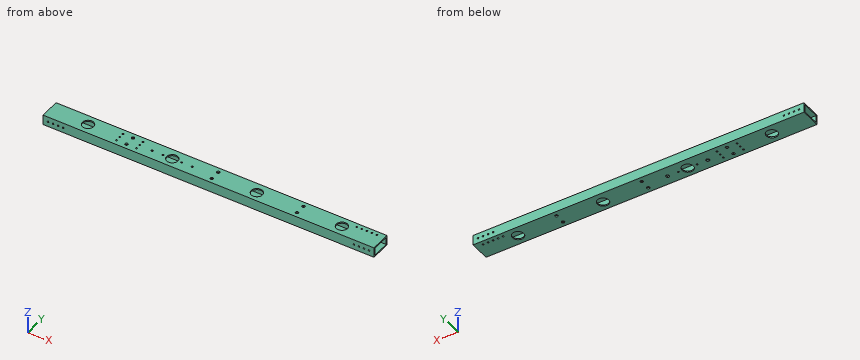
Autodesk Inventor part; units mm, degrees
ref_plane "YZ Plane" through (0, 0, 0) normal (1, 0, 0) x (0, 1, 0)
ref_plane "XZ Plane" through (0, 0, 0) normal (0, 1, 0) x (-1, 0, 0)
ref_plane "XY Plane" through (0, 0, 0) normal (0, 0, 1) x (1, 0, 0)
sketch "Sketch1" plane through (0, 0, 0) normal (0, 1, 0) x (-1, 0, 0)
  point P0 (0, 0)
sketch "Sketch2" plane through (0, 0, 0) normal (0, 0, 1) x (1, 0, 0)
  line L0 (0, 0) -> (838.2, 0)
  line L1 (838.2, 0) -> (838.2, 50.8)
  line L2 (838.2, 50.8) -> (0, 50.8)
  line L3 (0, 50.8) -> (0, 0)
  circle A0 centre (740.5688, 25.4) radius 14.2875
  circle A1 centre (97.6371, 25.4) radius 14.2875
  line L4 (0, 25.4) -> (838.2, 25.4) construction
  circle A2 centre (311.9438, 23.8125) radius 14.2875
  circle A3 centre (288.1313, 23.8125) radius 2.159
  circle A4 centre (335.7563, 23.8125) radius 2.159
  circle A5 centre (362.7438, 23.8125) radius 2.54
  circle A6 centre (261.1438, 23.8125) radius 2.54
  circle A7 centre (327.8188, 23.8125) radius 7.9375 construction
  line L5 (97.6371, 25.4) -> (97.6371, 90.8259)
  line L6 (740.5688, 25.4) -> (740.5688, 86.7676)
  line L7 (327.8188, 23.8125) -> (327.8188, 91.6838)
  circle A8 centre (526.2563, 23.8125) radius 14.2875
  line L8 (526.2563, 23.8125) -> (327.8188, 23.8125)
  line L9 (97.6371, 25.4) -> (97.6371, 0) construction
  line L10 (311.9438, 23.8125) -> (311.9438, 0) construction
  line L11 (526.2563, 23.8125) -> (526.2563, 0) construction
  line L12 (740.5688, 25.4) -> (740.5687, 0) construction
  line L13 (740.5687, 0) -> (526.2563, 0) construction
  line L14 (311.9438, 0) -> (355.3784, 0)
  line L15 (526.2563, 0) -> (311.9438, 0) construction
  line L16 (97.6371, 0) -> (311.9438, 0) construction
  line L17 (204.7904, 0) -> (204.7904, 50.8) construction
  line L18 (633.4125, 0) -> (633.4125, 50.8) construction
  line L19 (419.1, 0) -> (419.1, 50.8) construction
  line L20 (526.2563, 0) -> (419.1, 0) construction
  line L21 (0, 25.4) -> (0, 0) construction
  line L22 (0, 25.4) -> (0, 50.8) construction
  line L23 (0, 38.1) -> (838.2, 38.1) construction
  line L24 (0, 0) -> (0, 25.4) construction
  line L25 (0, 12.7) -> (838.2, 12.7) construction
  circle A9 centre (419.1, 38.1) radius 3.81
  circle A10 centre (419.1, 12.7) radius 3.81
  line L26 (311.9438, 23.8125) -> (526.2563, 23.8125)
  line L27 (419.1, 23.8125) -> (419.1, 31.9987)
  circle A11 centre (203.2, 38.1) radius 3.81
  circle A12 centre (203.2, 12.7) radius 3.81
  circle A13 centre (635, 38.1) radius 3.81
  circle A14 centre (635, 12.7) radius 3.81
  point P0 (190.5066, 50.8)
  dimension "d0" = 50.8
  dimension "d1" = 838.2
  dimension "d9" = 28.575
  dimension "d10" = 28.575
  dimension "d13" = 23.8125
  dimension "d14" = 23.8125
  dimension "d17" = 28.575
  dimension "d18" = 4.318
  dimension "d19" = 4.318
  dimension "d20" = 50.8
  dimension "d21" = 50.8
  dimension "d22" = 5.08
  dimension "d23" = 5.08
  dimension "d70" = 214.3125
  dimension "d72" = 28.575
  dimension "d73" = 214.3125
  dimension "d74" = 214.3125
  dimension "d99" = 7.62
  dimension "d100" = 7.62
  dimension "d113" = 419.1
  dimension "d114" = 1.5875
  dimension "d116" = 7.62
  dimension "d117" = 7.62
  dimension "d118" = 7.62
  dimension "d119" = 7.62
  dimension "d120" = 203.2
  dimension "d121" = 203.2
  dimension "d122" = 203.2
  dimension "d123" = 203.2
extrude "Extrusion1" add sketch "Sketch2" along normal blind 25.4 contours A0 | A8 | A5 L8 | L8 A5 | A4 L8 | L8 A4 | A2 | A1 | L3 L2 L1 L0 | A3 | A6 | A9 | A10 | A11 | A12 | A13 | A14
shell "Shell1" thickness 3.175 removed faces 2 at (0, 33.8667, 16.9333) at (838.2, 16.9333, 8.4667)
extrude "Extrusion2" cut sketch "Sketch2" along normal blind 174.9425 contours A0 | A8 | A5 L8 | L8 A5 | A4 L8 | L8 A4 | A2 | A1 | A3 | A6 | A9 | A10 | A11 | A12 | A13 | A14
sketch "Sketch3" plane through (0, 0, 0) normal (0, 0, -1) x (-1, 0, 0)
  circle A0 centre (-261.1438, 23.8125) radius 2.54
  circle A1 centre (-362.7438, 23.8125) radius 2.54
  circle A2 centre (-362.7438, 23.8125) radius 2.54
  circle A3 centre (-362.7438, 23.8125) radius 4.445
  circle A4 centre (-261.1438, 23.8125) radius 4.445
  point P0 (0, 0)
  dimension "d29" = 8.89
  dimension "d30" = 8.89
extrude "Extrusion3" cut sketch "Sketch3" against normal up to surface (22.225 mm away) contours A0 | A3 | A4
sketch "Sketch5" plane through (0, 50.8, 0) normal (0, 1, 0) x (1, 0, 0)
  point P0 (0, 0)
sketch "Sketch6" plane through (0, 50.8, 0) normal (0, 1, 0) x (1, 0, 0)
  point P0 (0, 0)
sketch "Sketch7" plane through (0, 50.8, 0) normal (0, 1, 0) x (1, 0, 0)
  line L0 (0, -22.225) -> (0, -3.175) construction
  line L1 (0, -12.7) -> (838.2, -12.7) construction
  line L2 (838.2, 0) -> (838.2, -25.4) construction
  circle A0 centre (0, -12.7) radius 2.0701
  circle A1 centre (12.7, -12.7) radius 2.0701
  circle A2 centre (25.4, -12.7) radius 2.0701
  circle A3 centre (38.1, -12.7) radius 2.0701
  circle A4 centre (50.8, -12.7) radius 2.0701
  line L3 (419.1, -12.7) -> (419.1, -25.4) construction
  circle A5 centre (419.1, -12.7) radius 2.0701
  circle A6 centre (431.8, -12.7) radius 2.0701
  circle A7 centre (444.5, -12.7) radius 2.0701
  circle A8 centre (457.2, -12.7) radius 2.0701
  circle A9 centre (406.4, -12.7) radius 2.0701
  circle A10 centre (419.1, -12.7) radius 2.0701
  circle A11 centre (431.8, -12.7) radius 2.0701
  circle A12 centre (444.5, -12.7) radius 2.0701
  circle A13 centre (393.7, -12.7) radius 2.0701
  circle A14 centre (406.4, -12.7) radius 2.0701
  circle A15 centre (419.1, -12.7) radius 2.0701
  circle A16 centre (431.8, -12.7) radius 2.0701
  circle A17 centre (381, -12.7) radius 2.0701
  circle A18 centre (393.7, -12.7) radius 2.0701
  circle A19 centre (406.4, -12.7) radius 2.0701
  circle A20 centre (419.1, -12.7) radius 2.0701
  circle A21 centre (825.5, -12.7) radius 2.0701
  circle A22 centre (812.8, -12.7) radius 2.0701
  circle A23 centre (800.1, -12.7) radius 2.0701
  circle A24 centre (787.4, -12.7) radius 2.0701
  point P0 (0, 0)
  dimension "d77" = 4.1402
  dimension "d80" = 12.7
  dimension "d85" = 4.1402
  dimension "d88" = 12.7
  dimension "d91" = 12.7
extrude "Extrusion5" cut sketch "Sketch7" against normal through all contours A1 | A2 | A3 | A4 | A21 | A22 | A23 | A24
sketch "Sketch8" plane through (0, 0, 25.4) normal (0, 0, 1) x (1, 0, 0)
  point P0 (0, 0)
sketch "Sketch9" plane through (0, 0, 25.4) normal (0, 0, 1) x (1, 0, 0)
  line L0 (0, 0) -> (838.2, 0)
  line L1 (838.2, 0) -> (819.15, 0)
  line L2 (819.15, 0) -> (819.15, 50.8)
  line L3 (838.2, 50.8) -> (0, 50.8)
  line L4 (819.15, 50.8) -> (819.15, 53.2892)
  line L5 (819.15, 53.2892) -> (819.15, 41.2718)
  line L6 (819.15, 53.2892) -> (819.15, 40.5892)
  line L7 (819.15, 40.5892) -> (806.45, 40.5892)
  circle A0 centre (819.15, 40.5892) radius 2.0701
  circle A1 centre (806.45, 40.5892) radius 2.0701
  circle A2 centre (793.75, 40.5892) radius 2.0701
  circle A3 centre (781.05, 40.5892) radius 2.0701
  circle A4 centre (768.35, 40.5892) radius 2.0701
  dimension "d124" = 19.05
  dimension "d125" = 2.4892
  dimension "d126" = 12.7
  dimension "d127" = 12.7
  dimension "d128" = 4.1402
  dimension "d131" = 12.7
extrude "Extrusion6" cut sketch "Sketch9" against normal through all
sketch "Sketch10" plane through (0, 0, 25.4) normal (0, 0, 1) x (1, 0, 0)
  line L0 (838.2, 50.8) -> (0, 50.8)
  line L1 (0, 50.8) -> (0, 38.1)
  line L2 (0, 47.625) -> (0, 3.175)
  line L3 (0, 38.1) -> (203.2, 38.1)
  circle A0 centre (203.2, 38.1) radius 2.0701
  circle A1 centre (215.9, 38.1) radius 2.0701
  circle A2 centre (228.6, 38.1) radius 2.0701
  circle A3 centre (241.3, 38.1) radius 2.0701
  circle A4 centre (190.5, 38.1) radius 2.0701
  circle A5 centre (203.2, 38.1) radius 2.0701
  circle A6 centre (215.9, 38.1) radius 2.0701
  circle A7 centre (228.6, 38.1) radius 2.0701
  circle A8 centre (177.8, 38.1) radius 2.0701
  circle A9 centre (190.5, 38.1) radius 2.0701
  circle A10 centre (203.2, 38.1) radius 2.0701
  circle A11 centre (215.9, 38.1) radius 2.0701
  circle A12 centre (165.1, 38.1) radius 2.0701
  circle A13 centre (177.8, 38.1) radius 2.0701
  circle A14 centre (190.5, 38.1) radius 2.0701
  circle A15 centre (203.2, 38.1) radius 2.0701
  circle A16 centre (165.1, 25.4) radius 2.0701
  circle A17 centre (177.8, 25.4) radius 2.0701
  circle A18 centre (190.5, 25.4) radius 2.0701
  circle A19 centre (203.2, 25.4) radius 2.0701
  circle A20 centre (215.9, 25.4) radius 2.0701
  circle A21 centre (228.6, 25.4) radius 2.0701
  circle A22 centre (241.3, 25.4) radius 2.0701
  circle A23 centre (165.1, 12.7) radius 2.0701
  circle A24 centre (177.8, 12.7) radius 2.0701
  circle A25 centre (190.5, 12.7) radius 2.0701
  circle A26 centre (203.2, 12.7) radius 2.0701
  circle A27 centre (215.9, 12.7) radius 2.0701
  circle A28 centre (228.6, 12.7) radius 2.0701
  circle A29 centre (241.3, 12.7) radius 2.0701
  circle A30 centre (165.1, 0) radius 2.0701
  circle A31 centre (177.8, 0) radius 2.0701
  circle A32 centre (190.5, 0) radius 2.0701
  circle A33 centre (203.2, 0) radius 2.0701
  circle A34 centre (215.9, 0) radius 2.0701
  circle A35 centre (228.6, 0) radius 2.0701
  circle A36 centre (241.3, 0) radius 2.0701
  point P0 (0, 0)
  dimension "d138" = 12.7
  dimension "d139" = 203.2
  dimension "d140" = 4.1402
  dimension "d143" = 12.7
  dimension "d146" = 12.7
  dimension "d151" = 12.7
extrude "Extrusion7" cut sketch "Sketch10" against normal through all contours A8 L3 | L3 A8 | A2 | A17 | A21 | A24 | A28
equation "\"d70\" = d73"
properties part number "Chassis side 1" material "Aluminum 6061"
Read the model definition and answer for the solid it produces. Units are mm, in the model's axes. Give positions to 0.01 mm unless a question says otherwise; leave off trailing zeros. Order: outer loops, then holes, each group sorted by start corner. A loop starts at its lowest first (then second) coordinate and runs counter-clockwise, first axis right, second up.
(1) Straight lines are drawn through the part: L1, parallel to Z at x = 373, y = 21.5 (3 decimals); L2, parallel to Y at x = 414, z = 12.5 (3 decimals); L3, parallel to Z at x = 800.1, y = 49.85. For each, find the intervals that lie inside material, in ascending order.
(2) Given pin 1 (8 mm diameter, centred on x = 261.14, y = 23.81, fed in from -Z) (3 decimals); pin 2 (2.5 mm diameter, centred on x = 12.7, z = 12.7, fed in from -Y), each flat-ended and moving along its own axis, determine where each tip first touches the part or whether it passes through.
(3) Find section A-A (x = 709). Give the vertices of the cut face in (y, z) (3 decimals), plus the area to 3 significant figures.
Result sheet:
1. L1: z = 0 to 3.175, 22.225 to 25.4
1. L2: y = 0 to 3.175, 47.625 to 50.8
1. L3: z = 0 to 10.63, 14.77 to 25.4
2. pin 1: stops at z = 22.225
2. pin 2: passes through
3. outline: (0, 0) - (50.8, 0) - (50.8, 25.4) - (0, 25.4) - close; hole (3.175, 3.175) - (47.625, 3.175) - (47.625, 22.225) - (3.175, 22.225) - close
3. area: 444 mm2
